from build123d import *

# Parameters (mm, degrees)
F0_W      = 50
F0_H      = 80
F1_DEPTH  = 6
F2_W      = 5
F2_H      = 60
F3_DEPTH  = 30
F4_R      = 29.99999
F5_DEPTH  = 40
F7_DEPTH  = 65
F8_W      = 25
F8_H      = 6
F9_DEPTH  = 115.9
F10_R     = 1.5
F11_DEPTH = 30.7


# Not quite as in the source:
# - a fillet or chamfer is up to 0.001 mm smaller than in the source, because OpenCascade refuses the exact size


with BuildPart() as f1:
    # F0 (on Top) → F1 (new body)
    with BuildSketch(Plane.XY):
        Rectangle(F0_W, F0_H)
    extrude(amount=F1_DEPTH)

    # F2 (on face) → F3 (join)
    with BuildSketch(Plane.XY.offset(6)):
        Rectangle(F2_W, F2_H)
        with Locations((-10, 0)):
            Rectangle(F2_W, F2_H)
        with Locations((10, 0)):
            Rectangle(F2_W, F2_H)
    extrude(amount=F3_DEPTH)

    # F4 (radius 30 in the source; OpenCascade refuses exactly that, so slightly less here)
    f4_edges = [f1.edges().sort_by_distance(p)[0] for p in [
        (10, 30, 36),
        (0, 30, 36),
        (-10, 30, 36),
        (-10, -30, 36),
        (0, -30, 36),
        (10, -30, 36),
    ]]
    fillet(f4_edges, radius=F4_R)

    # F5 (add): a face of the model
    f5_faces = [f1.faces().sort_by_distance(p)[0] for p in [
        (0, 0, 0),
    ]]
    extrude(f5_faces, amount=F5_DEPTH)

    # F6 (on face) → F7 (cut)
    with BuildSketch(Plane(origin=(-25, 0, 0), x_dir=(0, -1, 0), z_dir=(-1, 0, 0))):
        with BuildLine():
            Line((40, -40), (40, -17))
            ThreePointArc((40, -17), (0, -7.2132285382), (-40, -17))
            Line((-40, -17), (-40, -40))
            Line((-40, -40), (40, -40))
        make_face()
    extrude(amount=-F7_DEPTH, mode=Mode.SUBTRACT)

    # F8 (on face) → F9 (cut)
    with BuildSketch(Plane(origin=(0, 40, 0), x_dir=(-1, 0, 0), z_dir=(0, 1, 0))):
        with Locations((0, -2)):
            Rectangle(F8_W, F8_H)
    extrude(amount=-F9_DEPTH, mode=Mode.SUBTRACT)

    # F10 (on face) → F11 (cut)
    with BuildSketch(Plane(origin=(-12.5, 0, 0), x_dir=(0, -1, 0), z_dir=(-1, 0, 0))):
        with Locations((0, 28)):
            Circle(F10_R)
    extrude(amount=-F11_DEPTH, mode=Mode.SUBTRACT)


solid = f1.part
Read the model definition and answer for the solid it produces. Units are mm, in the model's axes. A direction names the side the tool comes from. Coordinates: 2 decimals unless noted, no trailing zeros. Write each loop counter-clockwise with the first axis right and the second up, starting at its lowest first coordinate (ties: lowest second). Pieces come first, ordered by that corner, then holes. Notation, with made-up numbers: M 59,76.5 L 97,76.5 A17 ccw 97,88.5 Z; hole C -13.75,-3.5 d4. An arc over 180 degrees is marked long. Use a Markdown table: item, result.
Q1. The part is cut by section D-D, the plane y = 33. Write down the section's boundary in (x, z), then the cut area to 3 significant figures.
Answer block:
| item | result |
|---|---|
| outline | M -25,-13.74 L 25,-13.74 L 25,6 L -25,6 Z; hole M -12.5,-5 L 12.5,-5 L 12.5,1 L -12.5,1 Z |
| area | 837 mm2 |
Q2. The part is cut by section C-C, the plane z = 11. Write down the section's boundary in (x, y), then the cut area to 3 significant figures.
Answer block:
| item | result |
|---|---|
| outline | M -12.5,-29.58 L -7.5,-29.58 L -7.5,29.58 L -12.5,29.58 Z; M -2.5,-29.58 L 2.5,-29.58 L 2.5,29.58 L -2.5,29.58 Z; M 7.5,-29.58 L 12.5,-29.58 L 12.5,29.58 L 7.5,29.58 Z |
| area | 887 mm2 |
Q3. Each of these flat-tipped pins is pushed along its axis until it touches: pin 1 Ø20 at (x, y) = (6, -1) entering from -Z; pin 2 Ø15 at (y, z) = (-4, 23.5) entering from -X; pin 3 Ø2 at (y, z) = (-28, 8.5) entering from +X. Where does it stop, or does it pass through?
Answer block:
| item | result |
|---|---|
| pin 1 | stops at z = -7.91 |
| pin 2 | stops at x = -12.5 |
| pin 3 | stops at x = 12.5 |
Q4. Determine the mould class of faces 4 (the face through (-10.035, 0.195, 29.487)), 5 (the face through (0.035, -21.445, 26.979)), 6 (the face through (12.5, 0, 17)) for opening direction Y: released by +Y, released by -Y, zero draft, split by the parting line, or undercut.
Answer block:
| item | result |
|---|---|
| face 4 | undercut |
| face 5 | released by -Y |
| face 6 | zero draft |
Q5. Which of the six approach directions +Z, -Z, +X, -X, +Y, -Y give full straight-line access (tool end or side, diameter ignored) to faces 1 (the face through (12.5, 1, -2)), 2 (the face through (-2.5, 0, 17)), 3 (the face through (-12.5, 0, 17))?
Answer block:
| item | result |
|---|---|
| face 1 | +Y, -Y |
| face 2 | +Z, +Y, -Y |
| face 3 | +Z, -X, +Y, -Y |
Q6. The part is cut by section A-A, the plane x = 11. Give the number of separate pieces and of enclosed holes in the cut face, then the cut area to 3 significant figures.
Answer block:
| item | result |
|---|---|
| separate pieces | 2 |
| enclosed holes | 1 |
| area | 2,240 mm2 |
Q7. The part is cut by section B-B, the plane x = -6. Write down the section's boundary in (y, z).
Answer block:
| item | result |
|---|---|
| outline | M -40,-17 A86.64 cw 40,-17 L 40,-5 L -40,-5 Z; M -40,1 L 40,1 L 40,6 L -40,6 Z |
Q8. Straight lines are drawn through the part: L1, parallel to Z at x = 9.4, y = 0; L2, parallel to X at y = -19, z = 17; L3, parallel to X at y = -29.5, z = -2. For each, find the intervals that lie inside material, in ascending order. Write a range as [from, to].
Answer block:
| item | result |
|---|---|
| L1 | z = [-7.21, -5], [1, 26.5], [29.5, 36] |
| L2 | x = [-12.5, -7.5], [-2.5, 2.5], [7.5, 12.5] |
| L3 | x = [-25, -12.5], [12.5, 25] |
